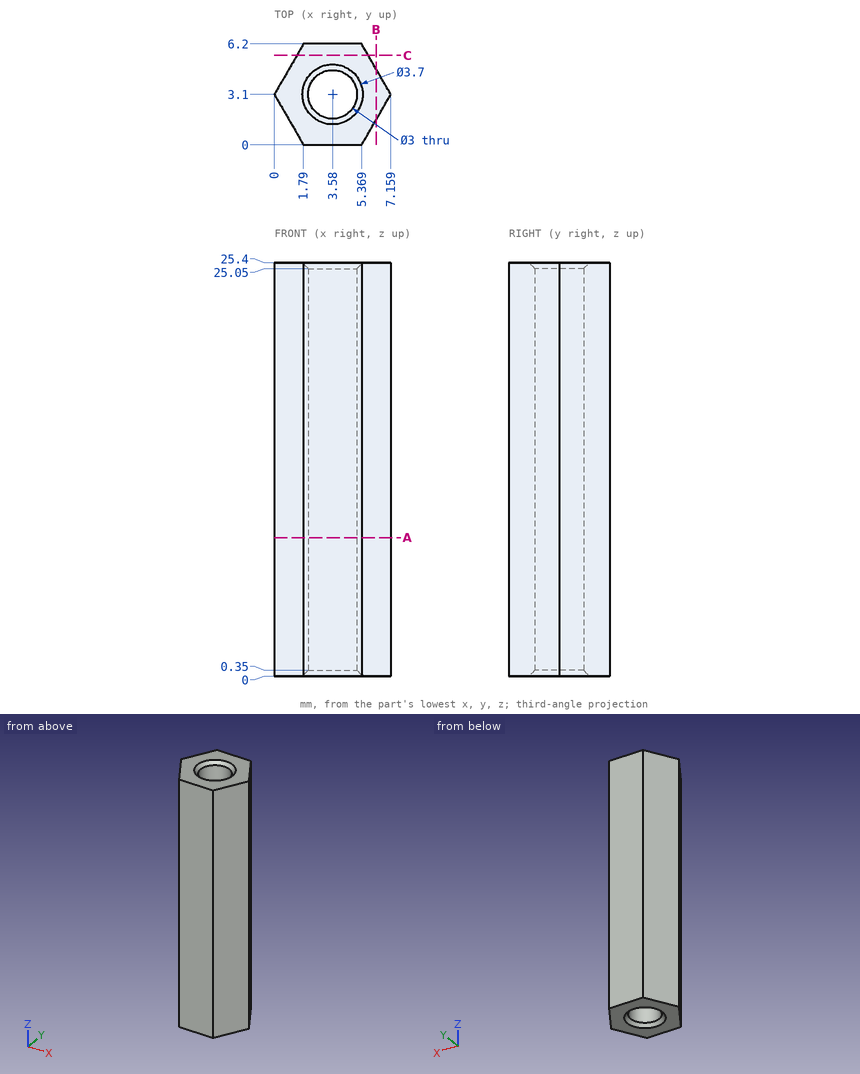
Check sheet for the drawn part. Datum: minimum x, y, z corner. Units: mm. Round coordinates to 2 decimals unless told otherwise and drop trailing zeros. Order: outer loops, then holes, each group sorted by start corner. A loop starts at its lowest first (then second) coordinate and runs counter-clockwise, first axis right, second up. Notation, with made-up numbers: (-28, 14.25) -> (11, 14.25) arc R14 ccw to (11, 32.25) -> close; hole circle Ø5 at (76, -29). An arc over 180 degrees is marked (long way). Return JSON: item names as keys, results as strings. Group by question number.
Q1. Gauge pin test, flat ends, axial feed: pin 1 (1.5 mm diameter, centred on x = 3, y = 1.5, fed in from -Z); pin 2 (1.5 mm diameter, centred on x = 1, z = 3, fed in from -Y); pin 3 (2.5 mm diameter, centred on x = 3.58, y = 3.1, fed in from -Z). Record the tip position at first contact, or that the pin passes through.
Q2. Material ranges on probe 1 along X at (y, z) = (1.75, 6.75) (1 decimal); probe 2 along Y at (x, z) = (2.75, 5.5); probe 3 along Y at (x, z) = (2.25, 15.75) (1 decimal), recorded low to high. Write a range as from..to.
Q3. Section check A-A, the plane z = 8.5. Record the boundary of the cut face in (x, y), plus the area to 3 significant figures.
Q4. Section check B-B, the plane x = 6.25. Record the boundary of the cut face in (y, z) (1 decimal).
Q5. Section check C-C, the plane y = 5.5. Record the boundary of the cut face in (x, z) (1 decimal).
Numbers:
{
 "1": {"pin 1": "z = 0", "pin 2": "y = 0.07", "pin 3": "through"},
 "2": {"probe 1": "0.8..2.9, 4.2..6.4", "probe 2": "0..1.85, 4.35..6.2", "probe 3": "0..2.4, 3.8..6.2"},
 "3": {"outline": "(0, 3.1) -> (1.79, 0) -> (5.37, 0) -> (7.16, 3.1) -> (5.37, 6.2) -> (1.79, 6.2) -> close; hole circle Ø3 at (3.58, 3.1)", "area": "26.2 mm^2"},
 "4": {"outline": "(1.5, 0) -> (4.7, 0) -> (4.7, 25.4) -> (1.5, 25.4) -> close"},
 "5": {"outline": "(1.4, 0) -> (5.8, 0) -> (5.8, 25.4) -> (1.4, 25.4) -> close"}
}
